Input: part model. Units: mm. Frame: model coordinates. A direction names the side the tool comes from. Round coordinates to 2 decimals unless told otherwise and drop trailing zeros. Loops run counter-clockwise (first coordinate to the right, second up) from the corner with the lowest first, then second, coordinate; pieces in that order, holes last. Notation, with made-up numbers: (60.5, 79) -> (98.5, 79) arc R14 cw to (98.5, 93) -> close; hole circle Ø6 at (-15.75, 0). An arc over 180 degrees is marked (long way). Answer as a JSON object with one key per item and string values. Group by question number.
Item 1: Section query B-B on x = 0. Return loops of the section in (y, z).
Item 2: Section query D-D on y = 43.5. Return loops of the section in (x, z).
Item 3: Material intervals for line 1 (Y direction, x = -110.5, z = -56); line 2 (Z direction, x = 126, y = 64); line 3 (Y direction, x = -15.5, z = 65.5), sorted ascending. Write a range as [from, to].
Item 4: Set-up query: faces 1 (the cylindrical face through (20.765, 81.874, 134.923)), 2 (the flat face through (107.5, 33, -1)), 3 (the flat face through (-1, 91, 94)). Return all of +Z, -Z, +X, -X, +Y, -Y with unobstructed straight access to the full face (end or side cutting, diameter ignored); none if empty.
Item 5: Section query C-C on z = -22. Return loops of the section in (x, y), and give its area (3 significant figures).
Item 6: Pin query (flat end, axial travel): pin 1 (4 mm diameter, centred on x = -127.5, y = 61, fed in from +Z); pin 2 (8 mm diameter, centred on x = 62.5, z = 34.5, fed in from -Y); pin 3 (6 mm diameter, centred on x = -121.5, y = 10.5, fed in from +Z). Return the tip coordinate at first contact, or that it passes through.
Item 7: Section query A-A on y = 14. Return loops of the section in (x, z), and give its area (3 significant figures).
Item 8: Draft query along Z for faces 4 (the cylindrical face through (-3.63, 35.99, 164.96)), 5 (the flat face through (2, 36, -155)), 6 (the flat face through (117, 14, -40)). Return one class per face: released by +Z, released by -Z, zero draft, split by the parting line, or undercut.
from build123d import *

# Parameters (mm, degrees)
BOSS_EXTRUDE1_DEPTH  = 73
SKETCH2_R            = 45
BOSS_EXTRUDE2_DEPTH  = 18
SKETCH3_W            = 20
SKETCH3_H            = 80
CUT_EXTRUDE2_DEPTH   = 27.5
SKETCH5_W            = 20
SKETCH5_H            = 40
LPATTERN2_COUNT      = 2
LPATTERN2_PITCH      = 180
LPATTERN2_COUNT_DIR2 = 2
LPATTERN2_PITCH_DIR2 = 200


with BuildPart() as part:
    # Sketch1 → Boss-Extrude1 (new body)
    with BuildSketch(Plane(origin=(0, 0, 0), x_dir=(1, 0, 0), z_dir=(0, 1, 0))):
        with BuildLine():
            ThreePointArc((-56.568542495, 155), (-135.201348942, 94.581156919), (-165, 0))
            ThreePointArc((-165, 0), (0, -165), (165, 0))
            ThreePointArc((165, 0), (135.201348942, 94.581156919), (56.568542495, 155))
            Line((56.568542495, 155), (-56.568542495, 155))
        make_face()
        with BuildLine():
            Line((-165, 155), (-165, 0))
            ThreePointArc((-165, 0), (-135.201348942, 94.581156919), (-56.568542495, 155))
            Line((-56.568542495, 155), (-165, 155))
        make_face()
        with BuildLine():
            ThreePointArc((56.568542495, 155), (135.201348942, 94.581156919), (165, 0))
            Line((165, 0), (165, 155))
            Line((165, 155), (56.568542495, 155))
        make_face()
    extrude(amount=BOSS_EXTRUDE1_DEPTH)

    # Sketch2 → Boss-Extrude2 (add)
    with BuildSketch(Plane(origin=(0, 73, 0), x_dir=(1, 0, 0), z_dir=(0, 1, 0))):
        with Locations((0, -95)):
            Circle(SKETCH2_R)
    extrude(amount=BOSS_EXTRUDE2_DEPTH)

    # Sketch4 one side → Revolve1 (revolve)
    with BuildSketch(Plane.XZ):
        with BuildLine():
            Line((-100, 100), (-80, 100))
            ThreePointArc((-80, 100), (-90, 110), (-100, 100))
        make_face()
    revolve1 = revolve(axis=Axis((-100, 0, 100), (1, 0, 0)))

    # Sketch3 → Cut-Extrude2 (cut)
    with BuildSketch(Plane.XZ):
        with Locations((-117.5, 0)):
            Rectangle(SKETCH3_W, SKETCH3_H)
        with Locations((117.5, 0)):
            Rectangle(SKETCH3_W, SKETCH3_H)
    extrude(amount=-CUT_EXTRUDE2_DEPTH, mode=Mode.SUBTRACT)

    # Sketch5 → Cut-Revolve2 (revolve, cut)
    with BuildSketch(Plane.XZ.offset(-27.5)):
        with Locations((-117.5, 20)):
            Rectangle(SKETCH5_W, SKETCH5_H)
        with Locations((117.5, 20)):
            Rectangle(SKETCH5_W, SKETCH5_H)
    revolve(axis=Axis((-127.5, 27.5, 0), (1, 0, 0)), mode=Mode.SUBTRACT)

    # LPattern2: Revolve1 2 × 2
    with Locations(*[(i * LPATTERN2_PITCH, 0, -j * LPATTERN2_PITCH_DIR2) for i in range(LPATTERN2_COUNT) for j in range(LPATTERN2_COUNT_DIR2) if (i, j) != (0, 0)]):
        add(revolve1)


solid = part.part
Solved:
{
 "1": {"outline": "(0, -155) -> (73, -155) -> (73, 50) -> (91, 50) -> (91, 140) -> (73, 140) -> (73, 165) -> (0, 165) -> close"},
 "2": {"outline": "(-165, -155) -> (165, -155) -> (165, 0) arc R165 ccw to (-165, 0) -> close; hole (-127.5, -36.66) -> (-107.5, -36.66) -> (-107.5, 36.66) -> (-127.5, 36.66) -> close; hole (107.5, -36.66) -> (127.5, -36.66) -> (127.5, 36.66) -> (107.5, 36.66) -> close"},
 "3": {"line 1": "[0, 73]", "line 2": "[-155, -16.36], [16.36, 106.53]", "line 3": "[0, 91]"},
 "4": {"face 1": "+Y", "face 2": "-Y", "face 3": "+Z, -Z, +X, -X, +Y"},
 "5": {"outline": "(-165, 0) -> (-127.5, 0) -> (-127.5, 60.91) -> (-107.5, 60.91) -> (-107.5, 0) -> (107.5, 0) -> (107.5, 60.91) -> (127.5, 60.91) -> (127.5, 0) -> (165, 0) -> (165, 73) -> (-165, 73) -> close", "area": "21,700 mm²"},
 "6": {"pin 1": "z = 107.12", "pin 2": "y = 0", "pin 3": "z = 114.82"},
 "7": {"outline": "(-165, -155) -> (165, -155) -> (165, 0) arc R165 ccw to (-165, 0) -> close; hole (-127.5, -40) -> (-107.5, -40) -> (-107.5, 40) -> (-127.5, 40) -> close; hole (107.5, -40) -> (127.5, -40) -> (127.5, 40) -> (107.5, 40) -> close", "area": "90,700 mm²"},
 "8": {"face 4": "released by +Z", "face 5": "released by -Z", "face 6": "undercut"}
}
